from build123d import *

# Parameters (mm, degrees)
SKETCH2_W           = 170
SKETCH2_H           = 220
BOSS_EXTRUDE1_DEPTH = 50
FILLET1_R           = 10
SKETCH3_W           = 150
SKETCH3_H           = 200
CUT_EXTRUDE1_DEPTH  = 50
SKETCH6_W           = 150
SKETCH6_H           = 200
BOSS_EXTRUDE2_DEPTH = 10
SKETCH7_W           = 170
SKETCH7_H           = 220
CUT_EXTRUDE3_DEPTH  = 30


with BuildPart() as part:
    # Sketch2 → Boss-Extrude1 (new body)
    with BuildSketch(Plane.XY):
        with Locations((33.670212766, 79.813829787)):
            Rectangle(SKETCH2_W, SKETCH2_H)
    extrude(amount=BOSS_EXTRUDE1_DEPTH)

    # Fillet1
    fillet1_edges = [part.edges().sort_by_distance(p)[0] for p in [
        (118.670212766, 79.813829787, 50),
        (33.670212766, 189.813829787, 50),
        (-51.329787234, 79.813829787, 50),
        (33.670212766, -30.186170213, 50),
    ]]
    fillet(fillet1_edges, radius=FILLET1_R)

    # Sketch3 → Cut-Extrude1 (cut)
    with BuildSketch(Plane(origin=(0, 0, 0), x_dir=(-1, 0, 0), z_dir=(0, 0, -1))):
        with Locations((-33.670212766, 79.813829787)):
            Rectangle(SKETCH3_W, SKETCH3_H)
    extrude(amount=-CUT_EXTRUDE1_DEPTH, mode=Mode.SUBTRACT)

    # Sketch6 → Boss-Extrude2 (add)
    with BuildSketch(Plane.XY.offset(40)):
        with Locations((33.670212766, 79.813829787)):
            Rectangle(SKETCH6_W, SKETCH6_H)
    extrude(amount=BOSS_EXTRUDE2_DEPTH)

    # Sketch7 → Cut-Extrude3 (cut)
    with BuildSketch(Plane.XY):
        with Locations((33.670212766, 79.813829787)):
            Rectangle(SKETCH7_W, SKETCH7_H)
    extrude(amount=CUT_EXTRUDE3_DEPTH, mode=Mode.SUBTRACT)


solid = part.part
Geometry: final body of the model. Coordinates: model frame, mm. A direction names the side the tool comes from. Coordinates: 2 decimals unless noted, no trailing zeros. Loops run counter-clockwise (first coordinate to the right, second up) from the corner with the lowest first, then second, coordinate; pieces in that order, holes last. Notation, with made-up numbers: (10, 53.25) - (53, 53.25) arc R25 ccw to (53, 72.25) - close; hole circle Ø4 at (65.25, 13.5). An arc over 180 degrees is marked (long way). One line per question, with ' | ' between items. Start each with the question number.
(1) Cut plane D-D on z = 44. Output: boundary loops of the cut face in (x, y).
(2) First-contact query: pin 1 (3 mm diameter, centred on y = 20.5, z = 48, fed in from -X); pin 2 (1.5 mm diameter, centred on x = 6.5, z = 47, fed in from +Y); pin 3 (8 mm diameter, centred on y = 88.5, z = 44.5, fed in from +X). Flat tips, straight axial feed; report the tip coordinate or a pass-through.
(3) Cut plane A-A on z = 34. Output: boundary loops of the cut face in (x, y).
(4) Cut plane C-C on x = 86.5. Output: boundary loops of the cut face in (y, z).
(5) Reachability of faces 4 (the flat face through (35, 179.814, 35)), 5 (the flat face through (32, -30.186, 35)) from +Z, -Z, +X, -X, +Y, -Y: full face, straight path, thin tool, end or side. Return the list, or none.
(6) Draft query along X for faces 1 (the flat face through (108.67, 78, 35)), 2 (the flat face through (-42, 88, 30)), 3 (the cylindrical face through (-48.48, 81.35, 46.99)). Return one class per face: +X half, -X half, draft (parallel to the pull), parting line (faces both ways), or undercut.
(7) Ray query, L1, parallel to X at y = 87.5, z = 38.25; L2, parallel to Y at x = -25, z = 34.25; L3, parallel to Z at x = 70, y = 180. Return the intervals inside material, ascending. Write a range as from..to.
(8) Cut plane B-B on y = 71. Output: boundary loops of the cut face in (x, z).
Here are the results:
1) outline: (-50.49, -29.35) - (117.84, -29.35) - (117.84, 188.98) - (-50.49, 188.98) - close
2) pin 1: x = -48.93 | pin 2: y = 187.62 | pin 3: x = 118.66
3) outline: (-51.33, -30.19) - (118.67, -30.19) - (118.67, 189.81) - (-51.33, 189.81) - close; hole (-41.33, -20.19) - (108.67, -20.19) - (108.67, 179.81) - (-41.33, 179.81) - close
4) outline: (-30.19, 30) - (-20.19, 30) - (-20.19, 40) - (179.81, 40) - (179.81, 30) - (189.81, 30) - (189.81, 40) arc R10 ccw to (179.81, 50) - (-20.19, 50) arc R10 ccw to (-30.19, 40) - close
5) face 4: -Z | face 5: +Z, -Z, +X, -X, -Y
6) face 1: undercut | face 2: draft | face 3: -X half
7) L1: -51.33..-41.33, 108.67..118.67 | L2: -30.19..-20.19, 179.81..189.81 | L3: 30..50
8) outline: (-51.33, 30) - (-41.33, 30) - (-41.33, 40) - (108.67, 40) - (108.67, 30) - (118.67, 30) - (118.67, 40) arc R10 ccw to (108.67, 50) - (-41.33, 50) arc R10 ccw to (-51.33, 40) - close
